Can you work these out from the drawing? Everything is in mm from the part's minimum corner. Round coordinates to 2 decimals unless told otherwise and drop trailing zeros. Order: outer loops, then holes, each group sorted by start corner. A loop starts at its lowest first (then second) coordinate and runs counter-clockwise, first axis right, second up. Notation, with made-up numbers: (60.25, -15) - (117.25, -15) arc R25 cw to (117.25, 20) - close; hole circle Ø6 at (-25, -31.5). An arc over 180 degrees is marked (long way). Answer as a JSON object with one key per item and string values.
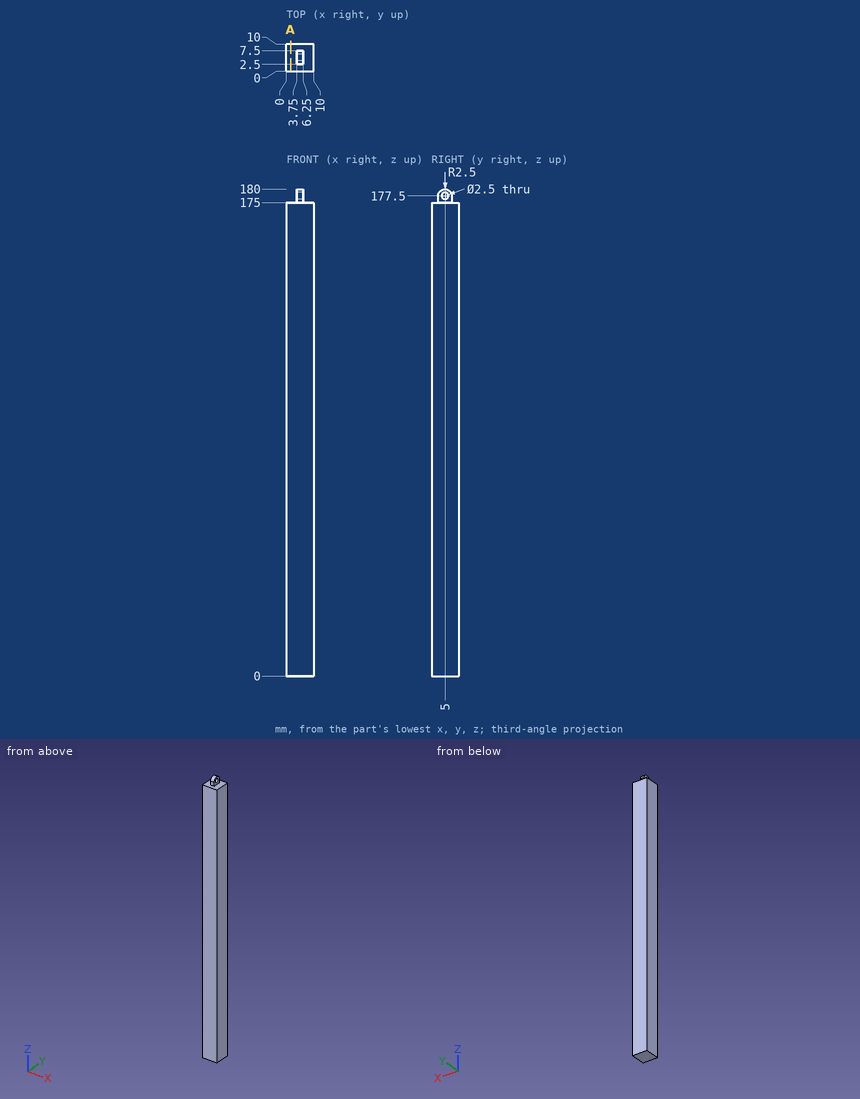
1. If I drill on L1, parallel to Y at x = 5.3, z = 177.5; L2, parallel to Z at x = 6, y = 4.75; L3, parallel to Z at x = 0.5, y = 1.5, over which ranges is the centre line in solid material (lowest first)? Write a range as [from, to].
Responses:
{"L1": "[2.5, 3.75], [6.25, 7.5]", "L2": "[0, 176.28], [178.72, 179.99]", "L3": "[0, 175]"}
2. For P1, Ø1.5, axis at y = 5.5, z = 177, coming from the -X side; P2, Ø4, axis at y = 4, z = 178, coming from the +X side; P3, Ø3, axis at x = 4, y = 2.5, coming from the +Z side, each with a flat end and sliding along its axis, tell me the tip position at first contact or that it passes through.
Responses:
{"P1": "x = 3.75", "P2": "x = 6.25", "P3": "z = 179.79"}
3. Imagine slicing it at A-A (x = 1.5). List the corners of the cut face in (y, z) for me.
Responses:
{"outline": "(0, 0) - (10, 0) - (10, 175) - (0, 175) - close"}
